Here's how the part is built. I have some questions about the finished solid (model axes, mm). A direction names the side the tool comes from. Coordinates: 2 decimals unless noted, no trailing zeros. Order: outer loops, then holes, each group sorted by start corner. A loop starts at its lowest first (then second) coordinate and runs counter-clockwise, first axis right, second up. Notation, with made-up numbers: (77, -6.75) - (103, -6.75) arc R22 ccw to (103, 24.25) - close; hole circle Ø5 at (-20, 25.25). An arc over 180 degrees is marked (long way). Answer in a Markdown table with one row per item. Add a question column.
Item 1: Will this pin go through, and if not, where does the flat tip stop? pin 1 Ø1.5 at (x, z) = (6.5, 1.5) entering from -Y.
Item 2: Thinking about a two-plate mould opening in X: for faces 3 (the flat face through (-40, 1, 4)), 4 (the cylindrical face through (21.123, 9.87, 3.944)), 5 (the flat face through (-1, 1, 0)), which applies, +X half, -X half, draft (parallel to the pull), parting line (faces both ways), or undercut?
Item 3: I want a section at A-A (x = -33). Please give me the cut outline in (y, z).
Item 4: If I drill on line 1 along Y through (x, z) = (32, 2); line 2 along Y through (x, z) = (-11, 6.5); line 3 along Y through (x, z) = (-21, 7.25), over which ranges is the centre line in solid material (lowest first)? Write a range as from..to.
Item 5: I want a section at B-B (z = 3.5). Count the separate pieces of the cut face and the enclosed holes in it, plus the area to 3 significant figures.
Item 6: On a 3-axis mill with a long thin cutter (end or side, diameter ignored), from which of +Z, -Z, +X, -X, +Y, -Y can I reach the whole of each face in a straight line? I mean faces 1 (the flat face through (-20, -56, 4)), 2 (the flat face through (-23, -90, 4)). Say none if no direction works.
```python
from build123d import *

# Parameters (mm, degrees)
F0_W     = 15
F0_H     = 8
F1_DEPTH = 8


with BuildPart() as f1:
    # F0 (on Top) → F1 (new body)
    with BuildSketch(Plane.XY):
        with BuildLine():
            Line((35, 90), (-35, 90))
            ThreePointArc((-35, 90), (-38.535534, 88.535534), (-40, 85))
            Line((-40, 85), (-40, -85))
            ThreePointArc((-40, -85), (-38.535534, -88.535534), (-35, -90))
            Line((-35, -90), (-10, -90))
            ThreePointArc((-10, -90), (0, -80), (10, -90))
            Line((10, -90), (35, -90))
            ThreePointArc((35, -90), (38.535534, -88.535534), (40, -85))
            Line((40, -85), (40, 85))
            ThreePointArc((40, 85), (38.535534, 88.535534), (35, 90))
        make_face()
        with Locations((-27.5, -56)):
            Rectangle(F0_W, F0_H, mode=Mode.SUBTRACT)
        with Locations((27.5, -56)):
            Rectangle(F0_W, F0_H, mode=Mode.SUBTRACT)
        with BuildLine():
            ThreePointArc((-25.263863, 50.035905), (-21.248199, 54.537215), (-16.024871, 57.554531))
            ThreePointArc((-16.024871, 57.554531), (-11.73955, 58.355979), (-7.412411, 57.824786))
            ThreePointArc((-7.412411, 57.824786), (-4.333461, 56.657266), (-1.206209, 55.626086))
            ThreePointArc((-1.206209, 55.626086), (0.532304, 55.237841), (2.270817, 55.626086))
            ThreePointArc((2.270817, 55.626086), (4.232387, 56.271409), (6.185894, 56.940745))
            ThreePointArc((6.185894, 56.940745), (9.185146, 57.975997), (12.318602, 58.474708))
            ThreePointArc((12.318602, 58.474708), (16.344444, 58.21585), (20.230889, 57.134203))
            ThreePointArc((20.230889, 57.134203), (24.03083, 54.814647), (27.014145, 51.510147))
            ThreePointArc((27.014145, 51.510147), (19.39754, 37.048347), (28.872508, 23.729888))
            ThreePointArc((28.872508, 23.729888), (26.721586, 18.523644), (23.953715, 13.617492))
            ThreePointArc((23.953715, 13.617492), (21.078874, 9.819793), (17.645785, 6.518109))
            ThreePointArc((17.645785, 6.518109), (15.624159, 5.522715), (13.403592, 5.139485))
            ThreePointArc((13.403592, 5.139485), (11.34891, 5.316623), (9.355833, 5.846472))
            ThreePointArc((9.355833, 5.846472), (7.255639, 6.665034), (5.120978, 7.388972))
            ThreePointArc((5.120978, 7.388972), (2.526786, 7.830283), (-0.104646, 7.817823))
            ThreePointArc((-0.104646, 7.817823), (-2.961809, 7.11564), (-5.716313, 6.081646))
            ThreePointArc((-5.716313, 6.081646), (-7.69726, 5.390047), (-9.773637, 5.088192))
            ThreePointArc((-9.773637, 5.088192), (-12.386956, 5.351298), (-14.690942, 6.612374))
            ThreePointArc((-14.690942, 6.612374), (-18.882856, 10.914265), (-22.349224, 15.81964))
            ThreePointArc((-22.349224, 15.81964), (-25.059935, 21.154457), (-27.020738, 26.808083))
            ThreePointArc((-27.020738, 26.808083), (-28.186358, 32.206624), (-28.448275, 37.723354))
            ThreePointArc((-28.448275, 37.723354), (-27.731572, 44.106062), (-25.263863, 50.035905))
        make_face(mode=Mode.SUBTRACT)
        with BuildLine():
            ThreePointArc((8.898433, 73.965858), (11.447708, 75.003195), (14.167834, 75.422469))
            ThreePointArc((14.167834, 75.422469), (14.204445, 73.96984), (14.167834, 72.517212))
            ThreePointArc((14.167834, 72.517212), (13.734786, 70.23514), (12.945735, 68.05047))
            ThreePointArc((12.945735, 68.05047), (11.497905, 65.553995), (9.692127, 63.302826))
            ThreePointArc((9.692127, 63.302826), (7.444453, 61.309154), (4.785833, 59.909686))
            ThreePointArc((4.785833, 59.909686), (2.503152, 59.320401), (0.145637, 59.324383))
            ThreePointArc((0.145637, 59.324383), (0.059444, 61.598708), (0.392238, 63.850205))
            ThreePointArc((0.392238, 63.850205), (2.121034, 67.770658), (4.769809, 71.138549))
            ThreePointArc((4.769809, 71.138549), (6.717839, 72.722006), (8.898433, 73.965858))
        make_face(mode=Mode.SUBTRACT)
    extrude(amount=F1_DEPTH)


solid = f1.part
```
Values follow:
| question | item | result |
|---|---|---|
| 1 | pin 1 | stops at y = -83.11 |
| 2 | face 3 | -X half |
| 2 | face 4 | undercut |
| 2 | face 5 | draft |
| 3 | outline | (-90, 0) - (-60, 0) - (-60, 8) - (-90, 8) - close; (-52, 0) - (90, 0) - (90, 8) - (-52, 8) - close |
| 4 | line 1 | y = -90..-60, -52..90 |
| 4 | line 2 | y = -90..5.08, 58.36..90 |
| 4 | line 3 | y = -90..-60, -52..13.71, 54.74..90 |
| 5 | separate pieces | 1 |
| 5 | enclosed holes | 4 |
| 5 | area | 11,400 mm^2 |
| 6 | face 1 | +Z, -Z |
| 6 | face 2 | +Z, -Z, +X, -X, -Y |
